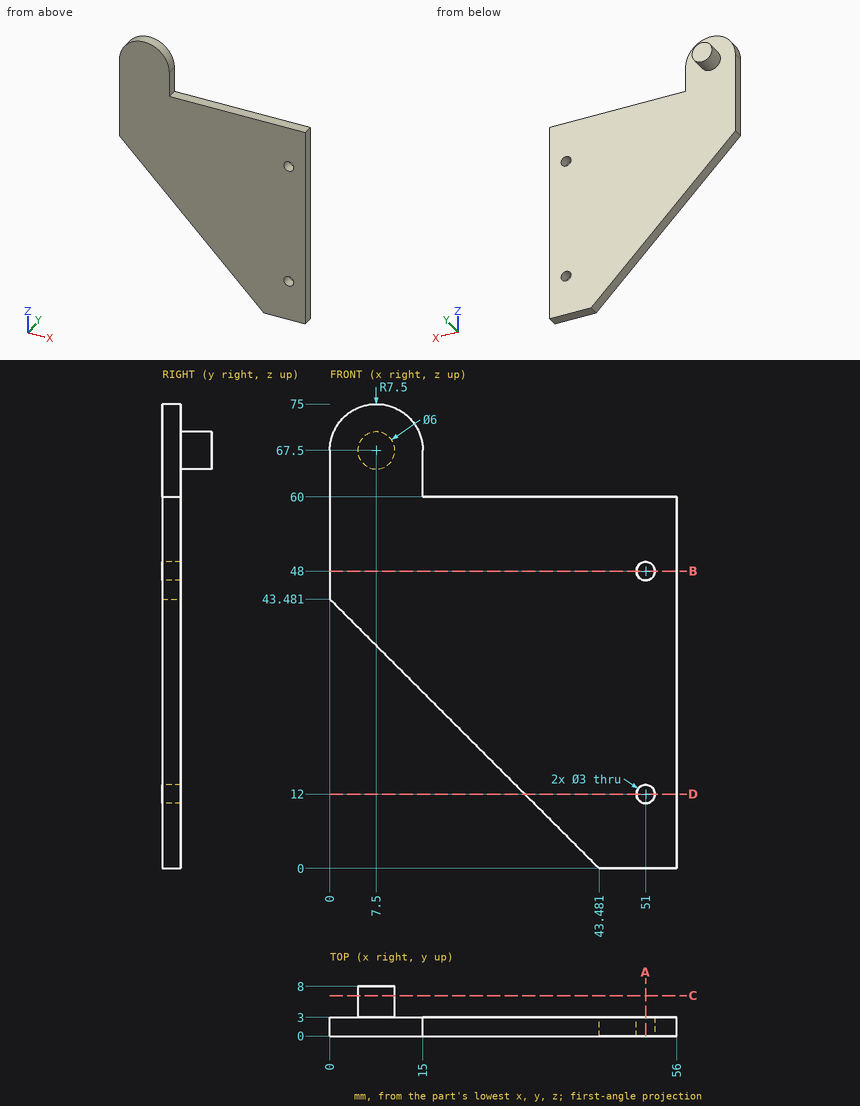
Verification items for this drawing (mm, ordinates from the low corner). Coordinates: 2 decimals unless noted, no trailing zeros. Order: outer loops, then holes, each group sorted by start corner. A loop starts at its lowest first (then second) coordinate and runs counter-clockwise, first axis right, second up. Notation, with made-up numbers: (63.25, -10.5) - (67.25, -10.5) arc R28 cw to (67.25, 27.5) - close; hole circle Ø4 at (-13, 65.5). An arc over 180 degrees is marked (long way). Answer as a JSON object with one key per item and string values. Group by question number.
Item 1: Sectioned sample at C-C, the plane y = 6.5. Record the cut outline in (x, z).
Item 2: Sectioned sample at D-D, the plane z = 12. Record the cut outline in (x, y).
Item 3: Depth check by flat-ended pin: pin 1 Ø2.5 at (x, z) = (51, 48) entering from +Y; pin 2 Ø17 at (x, z) = (14.5, 39.5) entering from +Y; pin 3 Ø1.5 at (x, y) = (42, 2) entering from +Z; pin 4 Ø2.5 at (y, z) = (2, 63.5) entering from +X. Enter the tip coordinate at first touch or a pass-through.
Item 4: Sectioned sample at B-B, the plane z = 48. Record the cut outline in (x, y), and give its area (3 significant figures).
Item 5: Scan lines: probe 1 along Z at (x, y) = (51, 1.3); probe 2 along Y at (x, z) = (36.5, 23); probe 3 along Z at (x, y) = (49, 1). Record each from-to range of solid material in increasing order.
Item 6: Sectioned sample at A-A, the plane x = 51. Record the cut outline in (y, z), and give its area (3 significant figures).
Resolved:
{
 "1": {"outline": "circle Ø6 at (7.5, 67.5)"},
 "2": {"outline": "(31.48, 0) - (49.5, 0) - (49.5, 3) - (31.48, 3) - close; (52.5, 0) - (56, 0) - (56, 3) - (52.5, 3) - close"},
 "3": {"pin 1": "through", "pin 2": "y = 3", "pin 3": "z = 60", "pin 4": "x = 15"},
 "4": {"outline": "(0, 0) - (49.5, 0) - (49.5, 3) - (0, 3) - close; (52.5, 0) - (56, 0) - (56, 3) - (52.5, 3) - close", "area": "159 mm^2"},
 "5": {"probe 1": "0 to 10.5, 13.5 to 46.5, 49.5 to 60", "probe 2": "0 to 3", "probe 3": "0 to 60"},
 "6": {"outline": "(0, 0) - (3, 0) - (3, 10.5) - (0, 10.5) - close; (0, 13.5) - (3, 13.5) - (3, 46.5) - (0, 46.5) - close; (0, 49.5) - (3, 49.5) - (3, 60) - (0, 60) - close", "area": "162 mm^2"}
}
